The model under review builds one solid part; all positions refer to its coordinate system, in mm. A direction names the side the tool comes from. Round coordinates to 2 decimals unless told otherwise and drop trailing zeros. Write each loop counter-clockwise with the first axis right and the second up, starting at its lowest first coordinate (ties: lowest second). Pieces come first, ordered by that corner, then holes. Notation, with made-up numbers: (79, 22.5) -> (129, 22.5) arc R6 ccw to (129, 32.5) -> close; hole circle Ø10 at (47, -10.75). An arc over 180 degrees is marked (long way). Return JSON: item names as keys, results as strings. Group by question number.
1. Tool access review of faces 1 (the flat face through (-25, 5, 0)), 2 (the cylindrical face through (-3.6, 17.6, -0.3)): name each direction out of +Z, -Z, +X, -X, +Y, -Y from which nothing blocks a thin tool from reaching the whole face with its end or side.
2. Mouldability with a two-part tool opening along Z and no side actions: class faces 3 (the conical face through (-0.86, 18.49, -9.55)), 4 (the flat face through (0, 5, 17.5)), 5 (the flat face through (0, 0, 0)), 6 (the flat face through (0, 10, -3)) as pulls with the +Z half, pulls with the -Z half, needs draft (parallel to the pull), parting line crosses it, or undercut.
3. Take a section at B-B, the plane y = 18.5. Write out the cut boundary in (x, z).
4. Take a section at D-D, the plane x = -16. Write out the cut boundary in (y, z), then the cut area to 3 significant figures.
5. Take a section at C-C, the plane z = 14. Write out the cut boundary in (x, y), then the cut area to 3 significant figures.
6. Clearance check with flat-ended pins moving along their axes: P1, Ø8, axis at y = 16, z = -11, coming from the -X side; P2, Ø2.5, axis at x = -1.5, z = -3, coming from the +Y side; P3, Ø5, axis at x = 10, y = 20.5, coming from the +Z side. State where each tip first meets the part, or that it passes through.
7. Take a section at A-A, the plane x = 0. Write out the cut boundary in (y, z).
8. For line 1 along Y through (x, z) = (16.5, -14); line 2 along Z through (x, y) = (0, 13.25); line 3 along Z through (x, y) = (0, 19.5), list the stretches that pass through material, from the lowest coordinate up. Write a range as from..to.
from build123d import *

# Parameters (mm, degrees)
SKETCH1_W           = 50
SKETCH1_H           = 35
BOSS_EXTRUDE1_DEPTH = 10
SKETCH2_R           = 7.5
BOSS_EXTRUDE2_DEPTH = 15
BOSS_EXTRUDE2_TAPER = 6
SKETCH3_R           = 4.5
CUT_EXTRUDE1_DEPTH  = 15
FILLET1_R           = 2


with BuildPart() as part:
    # Sketch1 → Boss-Extrude1 (new body)
    with BuildSketch(Plane(origin=(0, 0, 0), x_dir=(1, 0, 0), z_dir=(0, 1, 0))):
        Rectangle(SKETCH1_W, SKETCH1_H)
    extrude(amount=BOSS_EXTRUDE1_DEPTH)

    # Sketch2 → Boss-Extrude2 (add)
    with BuildSketch(Plane(origin=(0, 10, 0), x_dir=(1, 0, 0), z_dir=(0, 1, 0))):
        with Locations((0, 3)):
            Circle(SKETCH2_R)
    extrude(amount=BOSS_EXTRUDE2_DEPTH, taper=BOSS_EXTRUDE2_TAPER)

    # Sketch3 → Cut-Extrude1 (cut)
    with BuildSketch(Plane(origin=(0, 25, 0), x_dir=(1, 0, 0), z_dir=(0, 1, 0))):
        with Locations((0, 3)):
            Circle(SKETCH3_R)
    extrude(amount=-CUT_EXTRUDE1_DEPTH, mode=Mode.SUBTRACT)

    # Fillet1
    fillet1_edges = [part.edges().sort_by_distance(p)[0] for p in [
        (-7.5, 10, -3),
    ]]
    fillet(fillet1_edges, radius=FILLET1_R)


solid = part.part
Output:
{
 "1": {"face 1": "+Z, -Z, -X, +Y, -Y", "face 2": "+Y"},
 "2": {"face 3": "parting line crosses it", "face 4": "pulls with the +Z half", "face 5": "needs draft", "face 6": "undercut"},
 "3": {"outline": "circle Ø13.21 at (0, -3); hole circle Ø9 at (0, -3)"},
 "4": {"outline": "(0, -17.5) -> (10, -17.5) -> (10, 17.5) -> (0, 17.5) -> close", "area": "350 mm^2"},
 "5": {"outline": "(-25, 0) -> (25, 0) -> (25, 10) -> (-25, 10) -> close", "area": "500 mm^2"},
 "6": {"P1": "stops at x = -5.63", "P2": "stops at y = 10", "P3": "passes through"},
 "7": {"outline": "(0, -17.5) -> (10, -17.5) -> (10, -12.3) arc R2 cw to (11.79, -10.31) -> (25, -8.92) -> (25, -7.5) -> (10, -7.5) -> (10, 1.5) -> (25, 1.5) -> (25, 2.92) -> (11.79, 4.31) arc R2 cw to (10, 6.3) -> (10, 17.5) -> (0, 17.5) -> close"},
 "8": {"line 1": "y = 0..10", "line 2": "z = -10.16..-7.5, 1.5..4.16", "line 3": "z = -9.5..-7.5, 1.5..3.5"}
}
